```python
from build123d import *

# Parameters (mm, degrees)
BOSS_EXTRUDE2_DEPTH      = 27
SHELL5_DEPTH             = 17
BOSS_EXTRUDE3_START      = 10
BOSS_EXTRUDE3_DEPTH      = 10
SKETCH5_R                = 11
CUT_EXTRUDE2_DEPTH       = 87.360074687
BOSS_EXTRUDE4_DEPTH      = 37
BOSS_EXTRUDE5_DEPTH      = 3
BOSS_EXTRUDE5_DEPTH_BACK = 50
SKETCH10_R               = 2
CUT_EXTRUDE3_DEPTH       = 10
SKETCH11_W               = 121
SKETCH11_H               = 37
CUT_EXTRUDE4_DEPTH       = 92.526294036


# Read off the part's stored shape, not the designer's step: Shell5
with BuildPart() as part:
    # Sketch1 → Boss-Extrude2 (new body)
    with BuildSketch(Plane.XY):
        with BuildLine():
            ThreePointArc((20.25, 22.449944321), (-63.75, 0), (20.25, -22.449944321))
            ThreePointArc((20.25, -22.449944321), (41.25, 0), (20.25, 22.449944321))
        make_face()
    extrude(amount=BOSS_EXTRUDE2_DEPTH)

    # Shell5 outline → Shell5 (cut)
    with BuildSketch(Plane.XY):
        with BuildLine():
            ThreePointArc((14.25, -11.66190379), (31.25, 0), (14.25, 11.66190379))
            ThreePointArc((14.25, 11.66190379), (-53.75, 0), (14.25, -11.66190379))
        make_face()
    extrude(amount=SHELL5_DEPTH, mode=Mode.SUBTRACT)

    # Sketch4 → Boss-Extrude3 (add)
    with BuildSketch(Plane(origin=(0, 0, 0), x_dir=(-1, 0, 0), z_dir=(0, 0, -1)).offset(BOSS_EXTRUDE3_START)):
        with BuildLine():
            ThreePointArc((-20.25, 22.449944321), (-41.25, 0), (-20.25, -22.449944321))
            ThreePointArc((-20.25, -22.449944321), (63.75, 0), (-20.25, 22.449944321))
        make_face()
    extrude(amount=-BOSS_EXTRUDE3_DEPTH)

    # Sketch5 → Cut-Extrude2 (cut, through all)
    with BuildSketch(Plane(origin=(0, 0, -10), x_dir=(-1, 0, 0), z_dir=(0, 0, -1))):
        with Locations((-18.75, 0)):
            Circle(SKETCH5_R)
        with Locations((18.75, 0)):
            Circle(SKETCH5_R)
    extrude(amount=-CUT_EXTRUDE2_DEPTH, mode=Mode.SUBTRACT)

    # Sketch8 → Boss-Extrude4 (add)
    with BuildSketch(Plane(origin=(0, 0, -10), x_dir=(-1, 0, 0), z_dir=(0, 0, -1))):
        with BuildLine():
            Line((-41.25, 0), (-41.25, -50))
            Line((-41.25, -50), (63.75, -50))
            Line((63.75, -50), (63.75, 0))
            ThreePointArc((63.75, 0), (30.368950039, -43.474130239), (-20.25, -22.449944321))
            ThreePointArc((-20.25, -22.449944321), (-35.181676725, -15.370426149), (-41.25, 0))
        make_face()
    extrude(amount=-BOSS_EXTRUDE4_DEPTH)

    # Sketch9 → Boss-Extrude5 (add, two sides: drawn at the far end of the back side and taken through both)
    with BuildSketch(Plane(origin=(0, 0, 0), x_dir=(1, 0, 0), z_dir=(0, 1, 0)).offset(-BOSS_EXTRUDE5_DEPTH_BACK)):
        Polygon((-71.75, -27), (-58.75, -27), (-58.75, -8.5), (-58.75, 10), (-71.75, 10), align=None)
        Polygon((36.25, -8.5), (36.25, 10), (49.25, 10), (49.25, -27), (36.25, -27), align=None)
    extrude(amount=BOSS_EXTRUDE5_DEPTH + BOSS_EXTRUDE5_DEPTH_BACK)

    # Sketch10 → Cut-Extrude3 (cut)
    with BuildSketch(Plane(origin=(0, 3, 0), x_dir=(1, 0, 0), z_dir=(0, 1, 0))):
        with Locations(Location((-67.699944321, -8.5, 0), (0, 0, 270))):
            Circle(SKETCH10_R)
        with Locations(Location((45.199944321, -8.5, 0), (0, 0, 90))):
            Circle(SKETCH10_R)
    extrude(amount=-CUT_EXTRUDE3_DEPTH, mode=Mode.SUBTRACT)

    # Sketch11 → Cut-Extrude4 (cut, through all)
    with BuildSketch(Plane(origin=(0, 0, 0), x_dir=(1, 0, 0), z_dir=(0, 1, 0))):
        with Locations((-11.25, -8.5)):
            Rectangle(SKETCH11_W, SKETCH11_H)
    extrude(amount=-CUT_EXTRUDE4_DEPTH, mode=Mode.SUBTRACT)


solid = part.part
```
Model file for the job. Use its own axes, mm. A direction names the side the tool comes from. Give positions to 0.01 mm unless a question says otherwise; leave off trailing zeros. Write each loop counter-clockwise with the first axis right and the second up, starting at its lowest first coordinate (ties: lowest second). Pieces come first, ordered by that corner, then holes. Notation, with made-up numbers: M -32.5,70 L -4.5,70 A31 ccw -4.5,96 Z; hole C -5,34.5 d4. An arc over 180 degrees is marked long. Use a Markdown table: item, result.
1) Pin check, flat tips, straight feed: pin 1 (3 mm diameter, centred on x = 6, z = 5.5, fed in from +Y); pin 2 (6.5 mm diameter, centred on x = -69, z = 2.5, fed in from +Y); pin 3 (4 mm diameter, centred on y = 17, z = 19, fed in from -X). Stop position of each tip, or through.
Responses:
| item | result |
|---|---|
| pin 1 | stops at y = 38.53 |
| pin 2 | stops at y = 3 |
| pin 3 | stops at x = -61.18 |
2) Cut at D-D (y = 6). List the corners of the cut face in (x, z).
Responses:
| item | result |
|---|---|
| outline | M -63.35,-10 L -27.97,-10 L -27.97,0 L -53.23,0 L -53.23,17 L -27.97,17 L -27.97,27 L -63.35,27 Z; M -9.53,-10 L 9.53,-10 L 9.53,0 L -9.53,0 Z; M -9.53,17 L 9.53,17 L 9.53,27 L -9.53,27 Z; M 27.97,-10 L 40.44,-10 L 40.44,27 L 27.97,27 L 27.97,17 L 29.72,17 L 29.72,0 L 27.97,0 Z |
3) Pull direction X, two halves, no side cores. Call faces 4 (the flat face through (0, 0, -5)), 5 (the cylindrical face through (33.96, 16.58, 8.24)), 6 (the cylindrical face through (18.508, 10.997, -5.07)): +X half, -X half, draft (parallel to the pull), parting line (faces both ways), or undercut.
Responses:
| item | result |
|---|---|
| face 4 | draft |
| face 5 | +X half |
| face 6 | undercut |
4) Cut at A-A (z = -2). List the corners of the cut face in (x, y).
Responses:
| item | result |
|---|---|
| outline | M -71.75,0 L -29.75,0 A11 cw -7.75,0 L 7.75,0 A11 cw 29.75,0 L 49.25,0 L 49.25,3 L 41.05,3 A22.5 ccw 20.25,22.45 A45 ccw -63.65,3 L -71.75,3 Z |
5) Tool access for faces 1 (the cylindrical face through (-69.652, 1.521, 8.066)), 2 (the flat face through (-70, 3, 8)), 3 (the flat face through (-20, 18, 0)): list every direction of +Z, -Z, +X, -X, +Y, -Y with a clear straight run to the whole face (end or side of a thin tool).
Responses:
| item | result |
|---|---|
| face 1 | +Y, -Y |
| face 2 | +Z, -Z, -X, +Y |
| face 3 | -Y |
6) Cut at C-C (z = 8.5). List the corners of the cut face in (x, y), and give its area (3 significant figures).
Responses:
| item | result |
|---|---|
| outline | M -71.75,0 L -69.7,0 L -69.7,3 L -71.75,3 Z; M -65.7,0 L -53.75,0 A35 cw 14.25,11.66 A12.5 cw 31.25,0 L 43.2,0 L 43.2,3 L 41.05,3 A22.5 ccw 20.25,22.45 A45 ccw -63.65,3 L -65.7,3 Z; M 47.2,0 L 49.25,0 L 49.25,3 L 47.2,3 Z |
| area | 1,390 mm2 |
7) Cut at B-B (x = -18.75). List the corners of the cut face in (y, z).
Responses:
| item | result |
|---|---|
| outline | M 11,-10 L 45,-10 L 45,27 L 11,27 L 11,17 L 35,17 L 35,0 L 11,0 Z |
8) Drill centre lines: line 1 (Z direction, x = 5, y = 23.5); line 2 (X direction, y = 8.5, z = -4.5); line 3 (X direction, y = 2.25, z = 8.5). Where is each one in solid material? Low to high. Write a range as from..to.
Responses:
| item | result |
|---|---|
| line 1 | z = -10..0, 17..27 |
| line 2 | x = -62.94..-25.73, -11.77..11.77, 25.73..39.58 |
| line 3 | x = -71.75..-69.7, -65.7..-53.68, 31.05..43.2, 47.2..49.25 |
